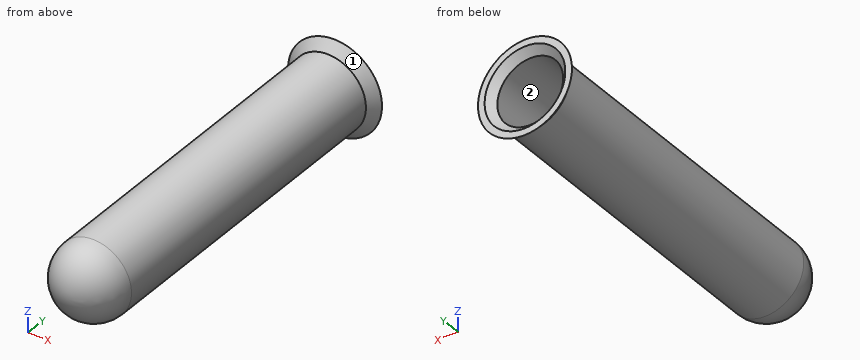
```python
from build123d import *

# Parameters (mm, degrees)
SHELL8_T = -1


with BuildPart() as part:
    # Sketch1 → Revolve2 (revolve)
    with BuildSketch(Plane.XY):
        with BuildLine():
            Line((0, 3.677706493), (10, 3.677706493))
            Line((10, 3.677706493), (8, 1.677706493))
            Line((8, 1.677706493), (8, -68.322293507))
            ThreePointArc((8, -68.322293507), (5.656854249, -73.979147757), (0, -76.322293507))
            Line((0, -76.322293507), (0, 3.677706493))
        make_face()
    revolve(axis=Axis((0, 3.677706493, 0), (0, -1, 0)))

    # Shell8
    shell8_openings = [part.faces().sort_by_distance(p)[0] for p in [
        (-10, 3.677706493, 0),
    ]]
    offset(amount=SHELL8_T, openings=shell8_openings, kind=Kind.INTERSECTION)


solid = part.part
```
Part model, mm, in its own coordinate system. Face numbers are marked on the shaded views. Give positions to 0.01 mm unless a question says otherwise; leave off trailing zeros. Write each loop counter-clockwise with the first axis right and the second up, starting at its lowest first coordinate (ties: lowest second). Pieces come first, ordered by that corner, then holes. Notation, with made-up numbers: (27.25, -31) -> (37.25, -31) arc R30 cw to (37.25, -9) -> close; hole circle Ø9 at (39, 28.5). An arc over 180 degrees is marked (long way). Put each result on its own line as item: value. Start each with the question number.
Item 1: Pin check, flat tips, straight feed: pin 1 Ø1.5 at (x, y) = (-4, -16) entering from +Z; pin 2 Ø8 at (x, y) = (-1, -14) entering from +Z; pin 3 Ø3 at (x, y) = (-8, -49.5) entering from +Z. Stop position of each tip, or through.
Item 2: Cut at C-C (y = -38). List the corners of the cut face in (x, z).
Item 3: Wall check: L1, parallel to Z at x = 0, y = -49; L2, parallel to X at y = -12.5, z = 3.25; L3, parallel to X at y = -2, z = -3.75. Give the ranges that are in metal, low to high. Write a range as [from, to].
Item 4: Pull direction Z, two halves, no side cores. Call the marked faces 1 and 2: pulls with the +Z half, pulls with the -Z half, needs draft (parallel to the pull), parting line crosses it, or undercut.
Item 5: Cut at A-A (x = 0). List the corners of the cut face in (y, z).
Item 6: Cut at B-B (z = 0). List the corners of the cut face in (x, y), then the cut area to 3 significant figures.
Answer list:
1. pin 1: stops at z = 7.31
1. pin 2: stops at z = 8
1. pin 3: stops at z = 4.66
2. outline: circle Ø16 at (0, 0); hole circle Ø14 at (0, 0)
3. L1: z = [-8, -7], [7, 8]
3. L2: x = [-7.31, -6.2], [6.2, 7.31]
3. L3: x = [-7.07, -5.91], [5.91, 7.07]
4. face 1: parting line crosses it
4. face 2: undercut
5. outline: (-68.32, -8) -> (1.68, -8) -> (3.68, -10) -> (3.68, -8.59) -> (2.09, -7) -> (-68.32, -7) arc R7 cw to (-68.32, 7) -> (2.09, 7) -> (3.68, 8.59) -> (3.68, 10) -> (1.68, 8) -> (-68.32, 8) arc R8 ccw to start
6. outline: (-10, 3.68) -> (-8, 1.68) -> (-8, -68.32) arc R8 ccw to (8, -68.32) -> (8, 1.68) -> (10, 3.68) -> (8.59, 3.68) -> (7, 2.09) -> (7, -68.32) arc R7 cw to (-7, -68.32) -> (-7, 2.09) -> (-8.59, 3.68) -> close
6. area: 169 mm2
